Geometry check sheet. Reference: drawing and pictorial views, mm from the part's lowest x, y, z. Give positions to 0.01 mm unless a question says otherwise; leave off trailing zeros. Write each loop counter-clockwise with the first axis right and the second up, starting at its lowest first coordinate (ties: lowest second). Pieces come first, ordered by that corner, then holes. Notation, with made-up numbers: (-13.5, 74) - (6.5, 74) arc R16 ccw to (6.5, 101) - close; hole circle Ø2 at (-32, -33). An arc over 180 degrees is marked (long way). Put each result on its own line as item: value.
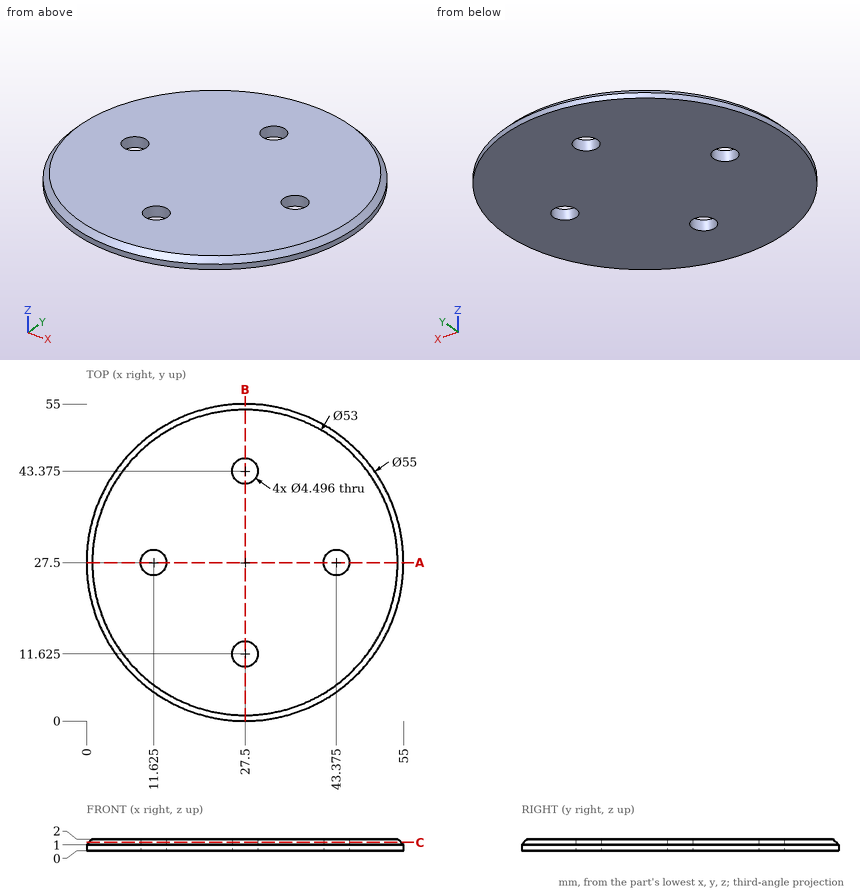
Q1. Section check C-C, the plane z = 1.4. Record the cut outline in (x, y) (1 decimal), plus the area to 3 significant figures.
Answers follow:
outline: circle Ø54.2 at (27.5, 27.5); hole circle Ø4.5 at (11.6, 27.5); hole circle Ø4.5 at (27.5, 11.6); hole circle Ø4.5 at (27.5, 43.4); hole circle Ø4.5 at (43.4, 27.5)
area: 2,240 mm2
Q2. Go/stop test with a flat-tipped pin: pin 1 Ø1 at (x, z) = (34.5, 1.5) entering from -Y. Record where the tip stops, or that it passes through.
Answers follow:
pin 1: stops at y = 0.89
Q3. Section check A-A, the plane y = 27.5. Record the cut outline in (x, z).
Answers follow:
outline: (0, 0) - (9.38, 0) - (9.38, 2) - (1, 2) - (0, 1) - close; (13.87, 0) - (41.13, 0) - (41.13, 2) - (13.87, 2) - close; (45.62, 0) - (55, 0) - (55, 1) - (54, 2) - (45.62, 2) - close
Q4. Scan lines: line 1 along Y through (x, z) = (27.5, 0.2); line 2 along Y through (x, z) = (27.5, 1.25); line 3 along Y through (x, z) = (42, 0.1). Record each from-to range of solid material in increasing order.
Answers follow:
line 1: y = 0 to 9.38, 13.87 to 41.13, 45.62 to 55
line 2: y = 0.25 to 9.38, 13.87 to 41.13, 45.62 to 54.75
line 3: y = 4.13 to 25.72, 29.28 to 50.87
